Geometry check sheet. Reference: the model listing, model coordinates, mm. A direction names the side the tool comes from. Give positions to 0.01 mm unless a question says otherwise; leave off trailing zeros. Loops run counter-clockwise (first coordinate to the right, second up) from the corner with the lowest first, then second, coordinate; pieces in that order, holes last. Notation, with made-up numbers: (-4, -21) - (33, -21) arc R27 cw to (33, 4) - close; hole circle Ø3 at (70.5, -0.5). An arc over 180 degrees is marked (long way). Use a Markdown table: item, result. Add a question column.
1. Draft check along X on faces 4 (the flat face through (141, 0, 4.5)), 5 (the flat face through (40, 0, 4.5)), 6 (the cylindrical face through (188, -6, 0)), 7 (the flat face through (195, 0, 0)). Enter one of: pulls with the +X half, pulls with the -X half, needs draft (parallel to the pull), parting line crosses it, or undercut.
2. Material ranges on L1, parallel to Y at x = 84, z = 0.5; L2, parallel to Z at x = 61.5, y = -0.25; L3, parallel to Y at x = 133, z = 4.75, recorded low to high.
3. Set-up check for faces 1 (the cylindrical face through (-7, -6, 0)), 2 (the flat face through (-14, 0, 0)), 3 (the flat face through (181, -4, -5)): record each of +Z, -Z, +X, -X, +Y, -Y from which the full face is reachable in a straight line by a thin tool's end or side.
4. Depth check by flat-ended pin: P1, Ø1.5, axis at x = 26.5, z = -0.5, coming from the -Y side; P2, Ø1.5, axis at x = 143, z = 4.5, coming from the -Y side; P3, Ø4, axis at x = 131, y = -5.5, coming from the -Z side; P4, Ø1.3, axis at x = 139, z = 5.5, coming from the +Y side. Enter the tip coordinate at first touch or a pass-through.
5. Cross-section at C-C on x = 5.5. Enter the section's corners in (y, z).
6. Cross-section at B-B on z = 0. Enter the section's corners in (x, y).
Autodesk Inventor part; units mm, degrees
ref_plane "YZ Plane" through (0, 0, 0) normal (1, 0, 0) x (0, 1, 0)
ref_plane "XZ Plane" through (0, 0, 0) normal (0, 1, 0) x (-1, 0, 0)
ref_plane "XY Plane" through (0, 0, 0) normal (0, 0, 1) x (1, 0, 0)
sketch "Sketch_1" plane through (0, 0, 0) normal (0, 0, 1) x (1, 0, 0)
  line L0 (195, 0) -> (-14, 0)
  line L1 (-14, 0) -> (-14, 5.5)
  line L2 (-14, 5.5) -> (-13.5, 6)
  line L3 (-13.5, 6) -> (-0.2, 6)
  arc A0 (-0.2, 6) -> (0, 6.2) centre (-0.2, 6.2) ccw
  line L4 (0, 6.2) -> (0, 7)
  line L5 (0, 7) -> (0.5, 7.5)
  line L6 (0.5, 7.5) -> (180.5, 7.5)
  line L7 (180.5, 7.5) -> (181, 7)
  line L8 (181, 7) -> (181, 6.2)
  arc A1 (181, 6.2) -> (181.2, 6) centre (181.2, 6.2) ccw
  line L9 (181.2, 6) -> (194.5, 6)
  line L10 (194.5, 6) -> (195, 5.5)
  line L11 (195, 5.5) -> (195, 0)
  line L12 (195, 0) -> (-14, 0)
revolve "Revolution1" add sketch "Sketch_1" angle 360 about axis through (195, 0, 0) along (1, 0, 0)
sketch "_____2" plane through (0, 0, 7.5) normal (0, 0, 1) x (1, 0, 0)
  arc A0 (32.5, 2.5) -> (32.5, -2.5) centre (32.5, 0) ccw
  line L0 (32.5, -2.5) -> (47.5, -2.5)
  arc A1 (47.5, -2.5) -> (47.5, 2.5) centre (47.5, 0) ccw
  line L1 (47.5, 2.5) -> (32.5, 2.5)
extrude "Extrusion1" cut sketch "_____2" against normal blind 3
sketch "_____6" plane through (0, 0, 7.5) normal (0, 0, 1) x (1, 0, 0)
  arc A0 (133.5, 2.5) -> (133.5, -2.5) centre (133.5, 0) ccw
  line L0 (133.5, -2.5) -> (148.5, -2.5)
  arc A1 (148.5, -2.5) -> (148.5, 2.5) centre (148.5, 0) ccw
  line L1 (148.5, 2.5) -> (133.5, 2.5)
extrude "Extrusion2" cut sketch "_____6" against normal blind 3
properties part number "NSFRQ15-181-F14-P12-T14-Q12-WKC30-C20-K30-E20_s"
Values found:
| question | item | result |
|---|---|---|
| 1 | face 4 | undercut |
| 1 | face 5 | undercut |
| 1 | face 6 | needs draft |
| 1 | face 7 | pulls with the +X half |
| 2 | L1 | y = -7.48 to 7.48 |
| 2 | L2 | z = -7.5 to 7.5 |
| 2 | L3 | y = -5.8 to -2.45, 2.45 to 5.8 |
| 3 | face 1 | -X |
| 3 | face 2 | +Z, -Z, -X, +Y, -Y |
| 3 | face 3 | +X |
| 4 | P1 | stops at y = -7.5 |
| 4 | P2 | stops at y = -6.5 |
| 4 | P3 | stops at z = -6.63 |
| 4 | P4 | stops at y = 5.72 |
| 5 | outline | circle Ø15 at (0, 0) |
| 6 | outline | (-14, -5.5) - (-13.5, -6) - (-0.2, -6) arc R0.2 cw to (0, -6.2) - (0, -7) - (0.5, -7.5) - (180.5, -7.5) - (181, -7) - (181, -6.2) arc R0.2 cw to (181.2, -6) - (194.5, -6) - (195, -5.5) - (195, 5.5) - (194.5, 6) - (181.2, 6) arc R0.2 cw to (181, 6.2) - (181, 7) - (180.5, 7.5) - (0.5, 7.5) - (0, 7) - (0, 6.2) arc R0.2 cw to (-0.2, 6) - (-13.5, 6) - (-14, 5.5) - close |
